Autodesk Inventor part; units mm, degrees
ref_plane "YZ Plane" through (0, 0, 0) normal (1, 0, 0) x (0, 1, 0)
ref_plane "XZ Plane" through (0, 0, 0) normal (0, 1, 0) x (-1, 0, 0)
ref_plane "XY Plane" through (0, 0, 0) normal (0, 0, 1) x (1, 0, 0)
sketch "スケッチ1" plane through (0, 0, 0) normal (0, 0, 1) x (1, 0, 0)
  line L0 (0, 0) -> (30, 0)
  line L1 (30, 0) -> (30, 40)
  line L2 (30, 40) -> (0, 40)
  line L3 (0, 40) -> (0, 0)
  point P0 (15, 20)
  dimension "d0" = 30
  dimension "d1" = 40
  dimension "d2" = 20
  dimension "d3" = 15
extrude "押し出し1" add sketch "スケッチ1" along normal blind 2
sketch "スケッチ2" plane through (0, 0, 2) normal (0, 0, 1) x (1, 0, 0)
  line L0 (30, 0) -> (30, 40)
  line L1 (30, 40) -> (0, 40)
  point P0 (0, 0)
  point P1 (15, 20)
  dimension "d6" = 15
  dimension "d7" = 20
hole "穴1" at (15, 20, 2) direction (0, 0, -1) diameter 3.242 end through all
sketch "スケッチ5" plane through (0, 0, 2) normal (0, 0, 1) x (1, 0, 0)
  line L0 (0, 40) -> (0, 0)
  line L1 (0, 0) -> (30, 0)
  line L2 (0, 2) -> (30, 2)
  line L3 (30, 2) -> (30, 0)
  line L4 (30, 0) -> (0, 0)
  line L5 (0, 0) -> (0, 2)
  dimension "d15" = 2
  dimension "d16" = 30
extrude "押し出し2" add sketch "スケッチ5" along normal blind 28
sketch "スケッチ10" plane through (0, 0, 0) normal (0, -1, 0) x (1, 0, 0)
  line L0 (11, 19) -> (19, 19)
  line L1 (19, 19) -> (19, 13)
  line L2 (19, 13) -> (11, 13)
  line L3 (11, 13) -> (11, 19)
  line L4 (30, 0) -> (30, 30)
  line L5 (0, 30) -> (30, 30)
  point P0 (0, 0)
  dimension "d32" = 8
  dimension "d33" = 11
  dimension "d34" = 11
  dimension "d35" = 6
extrude "押し出し6" cut sketch "スケッチ10" against normal blind 10
sketch "スケッチ11" plane through (0, 0, 0) normal (0, -1, 0) x (1, 0, 0)
  line L0 (11, 19) -> (19, 19)
  circle A0 centre (15, 19) radius 4
  line L1 (11, 13) -> (19, 13)
  circle A1 centre (15, 13) radius 4
  point P0 (0, 0)
  point P1 (12.3542, 16)
  point P2 (17.6458, 16)
extrude "押し出し7" cut sketch "スケッチ11" against normal blind 10 contours A0 L0 | A0 A1 L1
sketch "スケッチ12" plane through (0, 0, 0) normal (0, -1, 0) x (1, 0, 0)
  line L0 (11, 13) -> (19, 13)
  circle A0 centre (15, 13) radius 4
  point P0 (0, 0)
extrude "押し出し8" cut sketch "スケッチ12" against normal blind 10 contours L0 A0 picked at (13.7054, 12.6809)
properties part number "規定課題1"
Here's how the part is built. I have some questions about the finished solid (model axes, mm). A direction names the side the tool comes from. Coordinates: 2 decimals unless noted, no trailing zeros. Loops run counter-clockwise (first coordinate to the right, second up) from the corner with the lowest first, then second, coordinate; pieces in that order, holes last.
1. If we mould it in two halves opening along X, with no side actions, what happens to faces 4 (the cylindrical face through (15, 1, 9)), 5 (the flat face through (11, 21, 2)), 6 (the flat face through (30, 14.2, 1.6))? For each: pulls with the +X half, pulls with the -X half, needs draft (parallel to the pull), parting line crosses it, or undercut.
2. Imagine slicing it at A-A, the plane z = 17.25. Please give me the cut outline in (x, y).
3. Imagine slicing it at C-C, the plane x = 20.5. Please give me the cut outline in (y, z).
4. For faces 1 (the flat face through (15, 0, 8)), 2 (the flat face through (11, 1, 16)), 3 (the flat face through (8, 2, 16)), which set-ups out of +Z, -Z, +X, -X, +Y, -Y let a thin tool reach every point of the face, with its end or its side?
5. Imagine slicing it at D-D, the plane z = 12.25. Please give me the cut outline in (x, y).
6. For P1, Ø1, axis at y = 1, z = 16, coming from the -X side; P2, Ø12, axis at x = 15, z = 18, coming from the +Y side; P3, Ø1.5, axis at x = 13.5, y = 10, coming from the +Z side; P4, Ø1.5, axis at x = 17, z = 21, coming from the +Y side, each with a flat end and sliding along its axis, tell me the tip position at first contact or that it passes through.
7. Imagine slicing it at B-B, the plane x = 15. Please give me the cut outline in (y, z), and give its area (3 significant figures).
8. I need wall thicknesses on L1, parallel to X at y = 20, z = 0.4; L2, parallel to Y at x = 15, z = 1.65; L3, parallel to Z at x = 20.25, y = 24. Which ranges of each line are inside material? Lowest first, please.
Taken from the geometry:
1. face 4: undercut
1. face 5: needs draft
1. face 6: pulls with the +X half
2. outline: (0, 0) - (11, 0) - (11, 2) - (0, 2) - close; (19, 0) - (30, 0) - (30, 2) - (19, 2) - close
3. outline: (0, 0) - (40, 0) - (40, 2) - (2, 2) - (2, 30) - (0, 30) - close
4. face 1: +Z, -Z, +X, -X, -Y
4. face 2: +Y, -Y
4. face 3: +Z, +X, -X, +Y
5. outline: (0, 0) - (11.07, 0) - (11.07, 2) - (0, 2) - close; (18.93, 0) - (30, 0) - (30, 2) - (18.93, 2) - close
6. P1: stops at x = 0
6. P2: stops at y = 2
6. P3: stops at z = 2
6. P4: passes through
7. outline: (0, 0) - (18.38, 0) - (18.38, 2) - (2, 2) - (2, 9) - (0, 9) - close; (0, 23) - (2, 23) - (2, 30) - (0, 30) - close; (21.62, 0) - (40, 0) - (40, 2) - (21.62, 2) - close
7. area: 102 mm2
8. L1: x = 0 to 13.38, 16.62 to 30
8. L2: y = 0 to 18.38, 21.62 to 40
8. L3: z = 0 to 2
